Model file for the job. Use its own axes, mm. Coordinates: 2 decimals unless noted, no trailing zeros. Write each loop counter-clockwise with the first axis right and the second up, starting at its lowest first coordinate (ties: lowest second). Pieces come first, ordered by that corner, then holes. Notation, with made-up numbers: M 72.25,28.25 L 91.25,28.25 A19 ccw 91.25,33.25 Z; hole C -8.5,15.25 d4. An arc over 180 degrees is marked long. Put each result on its own line as item: value. Start each with the question number.
Q1. Cut at C-C (x = 12). Write the cut outline in (y, z).
Q2. Drop a flat-ended pin along its axis: pin 1 (1 mm diameter, centred on x = -25.5, z = 0, fed in from -Y). Give the stop position or say it passes through.
Q3. Drill centre lines: line 1 along Y through (x, z) = (0, 0.1); line 2 along Y through (x, z) = (27, -0.1); line 3 along Y through (x, z) = (-14.5, -0.3). Where is each one in solid material? Low to high.
Q4. Cut at D-D (y = 20.5). Write the cut outline in (x, z), then the cut area to 3 significant figures.
Q5. Cut at A-A (x = 0). Write the cut outline in (y, z).
Q6. Pull direction Y, two halves, no side cores. Call faces 1 (the cylindrical face through (-26.3, 25.45, -0.01)), 2 (the flat face through (-12.9, -28.5, -1)), 3 (the cylindrical face through (-0.537, -42.997, 0.014)): pulls with the +Y half, pulls with the -Y half, needs draft (parallel to the pull), parting line crosses it, or undercut.
```python
from build123d import *

# Parameters (mm, degrees)
SKETCH1_R           = 2
SKETCH1_R_2         = 31
BOSS_EXTRUDE1_DEPTH = 1


with BuildPart() as part:
    # Sketch1 → Boss-Extrude1 (new, symmetric)
    with BuildSketch(Plane.XY):
        with BuildLine():
            ThreePointArc((41.821047333, 10), (0, 43), (-41.821047333, 10))
            ThreePointArc((-41.821047333, 10), (-43, 0), (-41.821047333, -10))
            ThreePointArc((-41.821047333, -10), (-41.753494763, -10.278408199), (-41.684088814, -10.556360154))
            ThreePointArc((-41.684088814, -10.556360154), (0.263191219, -42.999194532), (41.810188324, -10.045304987))
            ThreePointArc((41.810188324, -10.045304987), (41.815623964, -10.022653964), (41.821047333, -10))
            ThreePointArc((41.821047333, -10), (43, 0), (41.821047333, 10))
        make_face()
        with Locations((-27.223611076, -27.223611076)):
            Circle(SKETCH1_R, mode=Mode.SUBTRACT)
        with Locations((0, -38.5)):
            Circle(SKETCH1_R, mode=Mode.SUBTRACT)
        with Locations((27.223611076, -27.223611076)):
            Circle(SKETCH1_R, mode=Mode.SUBTRACT)
        with Locations((-38.5, 0)):
            Circle(SKETCH1_R, mode=Mode.SUBTRACT)
        with Locations((-27.223611076, 27.223611076)):
            Circle(SKETCH1_R, mode=Mode.SUBTRACT)
        Circle(SKETCH1_R_2, mode=Mode.SUBTRACT)
        with Locations((38.5, 0)):
            Circle(SKETCH1_R, mode=Mode.SUBTRACT)
        with Locations((27.223611076, 27.223611076)):
            Circle(SKETCH1_R, mode=Mode.SUBTRACT)
        with Locations((0, 38.5)):
            Circle(SKETCH1_R, mode=Mode.SUBTRACT)
    extrude(amount=BOSS_EXTRUDE1_DEPTH, both=True)


solid = part.part
```
Computed values:
1. outline: M -41.29,-1 L -28.58,-1 L -28.58,1 L -41.29,1 Z; M 28.58,-1 L 41.29,-1 L 41.29,1 L 28.58,1 Z
2. pin 1: y = -34.99
3. line 1: -43 to -40.5, -36.5 to -31, 31 to 36.5, 40.5 to 43
3. line 2: -33.47 to -29.21, -25.24 to -15.23, 15.23 to 25.24, 29.21 to 33.47
3. line 3: -40.48 to -27.4, 27.4 to 40.48
4. outline: M -37.8,-1 L -23.25,-1 L -23.25,1 L -37.8,1 Z; M 23.25,-1 L 37.8,-1 L 37.8,1 L 23.25,1 Z
4. area: 58.2 mm2
5. outline: M -43,-1 L -40.5,-1 L -40.5,1 L -43,1 Z; M -36.5,-1 L -31,-1 L -31,1 L -36.5,1 Z; M 31,-1 L 36.5,-1 L 36.5,1 L 31,1 Z; M 40.5,-1 L 43,-1 L 43,1 L 40.5,1 Z
6. face 1: undercut
6. face 2: needs draft
6. face 3: pulls with the -Y half
